Here's how the part is built. I have some questions about the finished solid (model axes, mm). Round coordinates to 2 decimals unless told otherwise and drop trailing zeros. Order: outer loops, then holes, each group sorted by start corner. A loop starts at its lowest first (then second) coordinate and runs counter-clockwise, first axis right, second up. Notation, with made-up numbers: M -21.5,-6 L -16.5,-6 A24 ccw -16.5,30 Z; hole C -29,39.25 d6. An arc over 180 degrees is marked long. Write item = value, one per line. Start each with the question number.
Item 1: I'm going to push a flat-ended pin straight in: P1, Ø2, axis at x = 44.5, y = 24.5, coming from the +Z side. Where does the tip first touch, or does it pass through?
Item 2: Please list where these lines run through material, in increasing order: L1, parallel to Y at x = 23.5, z = -6.5; L2, parallel to Z at x = 29, y = 34.5; L3, parallel to Y at x = 43.5, z = -13.5.
Item 3: I want a section at C-C, the plane z = -22. List the corners of the cut face in (x, y) for me.
Item 4: I want a section at D-D, the plane x = 19. List the corners of the cut face in (y, z) for me.
Autodesk Inventor part; units mm, degrees
ref_plane "工作平面1" through (20, 40, -20) normal (0.5747, 0.7663, 0.2873) x (-0.4472, 0, 0.8944)
ref_plane "工作平面2" through (50, 40, -30) normal (-0.2294, -0.6882, -0.6882) x (0, -0.7071, 0.7071)
ref_plane "YZ Plane" through (0, 0, 0) normal (1, 0, 0) x (0, 1, 0)
sketch "草圖1" plane through (0, 0, 0) normal (0, 1, 0) x (-1, 0, 0)
  line L0 (0, 0) -> (-50, 0)
  line L1 (-50, 0) -> (-50, -40)
  line L2 (-50, -40) -> (0, -40)
  line L3 (0, -40) -> (0, 0)
  dimension "d0" = 40
  dimension "d1" = 50
extrude "擠出1" add sketch "草圖1" along normal blind 40
sketch "草圖2" plane through (0, 0, 0) normal (0, 0, 1) x (1, 0, 0)
  line L0 (50, 10) -> (10, 40)
  line L1 (0, 40) -> (50, 40)
  line L2 (50, 0) -> (50, 40)
  point P0 (0, 0)
  dimension "d4" = 30
  dimension "d5" = 40
sketch "草圖3" plane through (0, 40, 0) normal (0, 1, 0) x (1, 0, 0)
  line L0 (0, 0) -> (50, 0)
  line L1 (50, 0) -> (50, 40)
  point P0 (20, 20)
  dimension "d6" = 20
  dimension "d7" = 30
ref_plane "工作平面1" through (20, 40, -20) normal (0.5747, 0.7663, 0.2873) x (-0.4472, 0, 0.8944)
sketch "草圖4" plane through (20, 40, -20) normal (0.5747, 0.7663, 0.2873) x (-0.4472, 0, 0.8944)
  line L0 (0, 0) -> (4.4721, 46.6905)
  line L1 (4.4721, 46.6905) -> (47.828, 42.5377)
  line L2 (47.828, 42.5377) -> (43.3559, -4.1527)
  line L3 (43.3559, -4.1527) -> (0, 0)
  point P0 (26.8328, 18.8475)
extrude "擠出2" cut sketch "草圖4" along normal blind 40
sketch "草圖5" plane through (50, 0, 0) normal (1, 0, 0) x (0, 0, -1)
  line L0 (2.1429, 40) -> (0, 10)
  line L1 (0, 10) -> (30, 40)
  line L2 (40, 40) -> (0, 40)
  point P0 (0, 0)
  dimension "d10" = 30
ref_plane "工作平面2" through (50, 40, -30) normal (-0.2294, -0.6882, -0.6882) x (0, -0.7071, 0.7071)
sketch "草圖6" plane through (50, 40, -30) normal (-0.2294, -0.6882, -0.6882) x (0, -0.7071, 0.7071)
  line L0 (7.0711, 30.8221) -> (19.698, 4.519)
  line L1 (19.698, 4.519) -> (42.4264, 0)
  line L2 (7.0711, 30.8221) -> (42.4264, 0)
  line L3 (42.4264, 0) -> (18.1406, -27.8578)
  line L4 (18.1406, -27.8578) -> (-17.2148, 2.9643)
  line L5 (-17.2148, 2.9643) -> (7.0711, 30.8221)
  point P0 (49.4975, 47.0442)
extrude "擠出3" cut sketch "草圖6" against normal blind 40
properties part number "24"
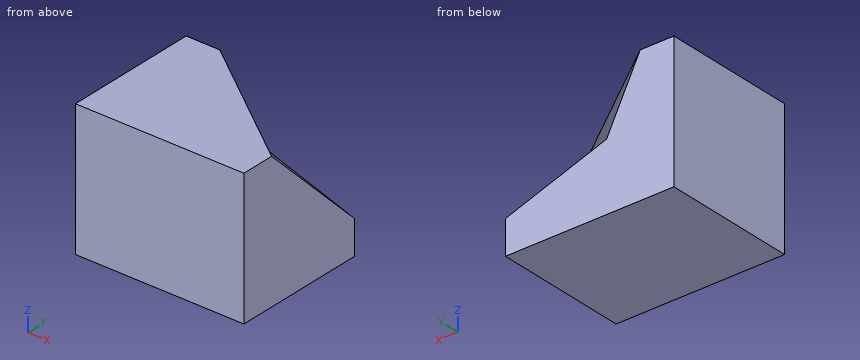
Filled in:
q1.P1 = -11.62
q2.L1 = 0 to 32.31
q2.L2 = -40 to -17.5
q2.L3 = 0 to 25.66
q3.outline = M 0,0 L 50,0 L 50,32 L 25.99,40 L 0,40 Z
q4.outline = M 0,-40 L 40,-40 L 40,-18.01 L 33.25,0 L 0,0 Z
